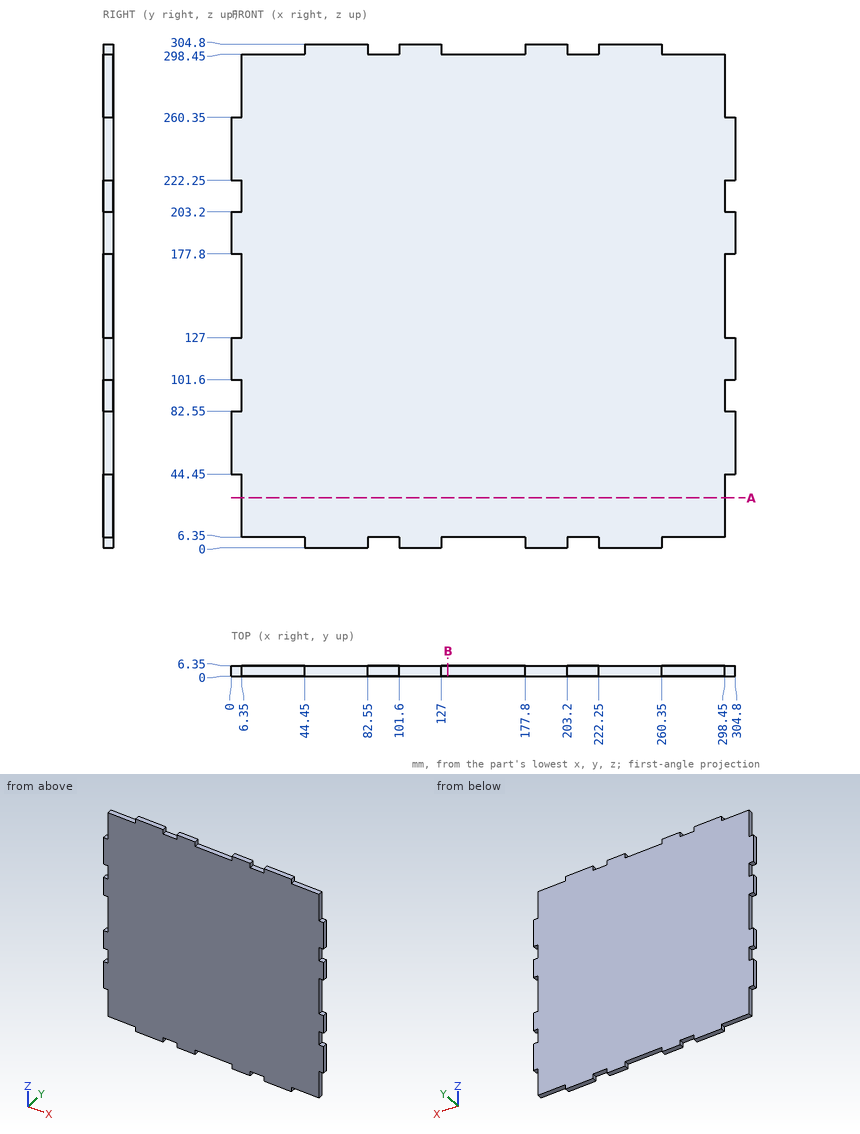
Job drawing, mm, ordinate dimensions from the low corner. One solid piece. Round coordinates to 2 decimals unless told otherwise and drop trailing zeros. Loops run counter-clockwise (first coordinate to the right, second up) from the corner with the lowest first, then second, coordinate; pieces in that order, holes last. Notation, with made-up numbers: (40, 89.5) -> (50, 89.5) arc R22 cw to (50, 124.5) -> close; hole circle Ø2 at (37, 74). An arc over 180 degrees is marked (long way). Use a Markdown table: item, result.
1) Probe line 1 (X direction, y = 1, z = 97). List the from-to ranges inside material, lowest first. Write a range as [from, to].
The answers:
| item | result |
|---|---|
| line 1 | x = [6.35, 298.45] |
2) Cut at B-B, the plane x = 131. List the corners of the cut face in (y, z).
The answers:
| item | result |
|---|---|
| outline | (0, 6.35) -> (6.35, 6.35) -> (6.35, 298.45) -> (0, 298.45) -> close |
3) Cut at A-A, the plane z = 30. List the corners of the cut face in (x, y).
The answers:
| item | result |
|---|---|
| outline | (6.35, 0) -> (298.45, 0) -> (298.45, 6.35) -> (6.35, 6.35) -> close |
4) Drop flat-ended pins along their axis: pin 1 Ø3 at (x, y) = (300, 1.5) entering from -Z; pin 2 Ø2 at (x, y) = (94, 4.5) entering from +Z; pin 3 Ø1.9 at (x, y) = (1.5, 4.5) entering from +Z. Give the stop position or say it passes through.
The answers:
| item | result |
|---|---|
| pin 1 | stops at z = 44.45 |
| pin 2 | stops at z = 298.45 |
| pin 3 | stops at z = 260.35 |
